For this review, use the dimensioned drawing (mm, ordinates from the lowest corner) and the shaded views. A direction names the side the tool comes from. Coordinates: 2 decimals unless noted, no trailing zeros. Write each loop counter-clockwise with the first axis right and the second up, starting at its lowest first coordinate (ties: lowest second). Pieces come first, ordered by that corner, then holes. Notation, with made-up numbers: M 23,67.5 L 77,67.5 A26 ccw 77,85.5 Z; hole C -29.75,50.5 d10. An arc over 180 degrees is marked long. Return JSON: item names as keys, results as strings.
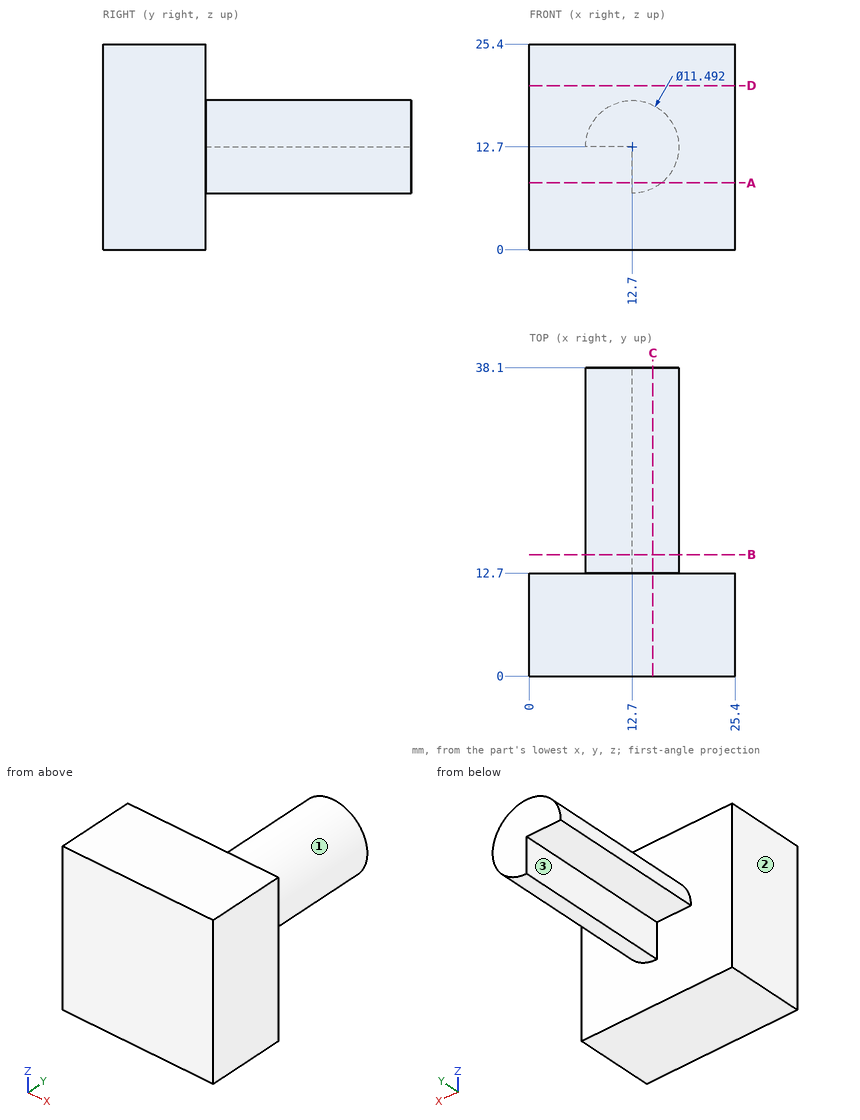
1. For the marked faces 1, 2 and 3, list the 3-axis set-ups (+Z, -Z, +X, -X, +Y, -Y) from which the entire face can be reached by the end or side of a thin tool; tool diameter is ignored.
Checks:
{"face 1": "+Y", "face 2": "+Z, -Z, -X, +Y, -Y", "face 3": "-Z, -X, +Y"}
2. We need section A-A (z = 8.25). State the section outline as (x, y) points (3 decimals), plus the area to 3 significant figures.
Checks:
{"outline": "M 0,0 L 25.4,0 L 25.4,12.7 L 16.335,12.7 L 16.335,38.1 L 12.7,38.1 L 12.7,12.7 L 0,12.7 Z", "area": "415 mm2"}
3. Clearance check with flat-ended pins moving along their axes: pin 1 Ø12 at (x, y) = (6.5, 28.5) entering from -Z; pin 2 Ø1 at (x, z) = (16.5, 19) entering from +Y; pin 3 Ø3 at (y, z) = (25.5, 9.5) entering from -X. State where each tip first meets the part, or that it passes through.
Checks:
{"pin 1": "z = 12.7", "pin 2": "y = 12.7", "pin 3": "x = 12.7"}
4. We need section D-D (z = 20.25). State the section outline as (x, y) points.
Checks:
{"outline": "M 0,0 L 25.4,0 L 25.4,12.7 L 0,12.7 Z"}
5. We need section B-B (y = 15). State the section outline as (x, z) points.
Checks:
{"outline": "M 6.95,12.7 L 12.7,12.7 L 12.7,6.95 A5.75 ccw long Z"}
6. We need section C-C (x = 15.25). State the section outline as (y, z) points, plus the area to 3 significant figures.
Checks:
{"outline": "M 0,0 L 12.7,0 L 12.7,7.55 L 38.1,7.55 L 38.1,17.85 L 12.7,17.85 L 12.7,25.4 L 0,25.4 Z", "area": "584 mm2"}
7. Wall thickness on L1, parallel to Z at x = 13, y = 29; L2, parallel to Y at x = 3, z = 19; L3, parallel to X at y = 29.5, z = 7.5 (1 decimal): over which ranges is each line inside the solid? List them lowest first. Write a range as from..to.
Checks:
{"L1": "6.96..18.44", "L2": "0..12.7", "L3": "12.7..15.1"}
